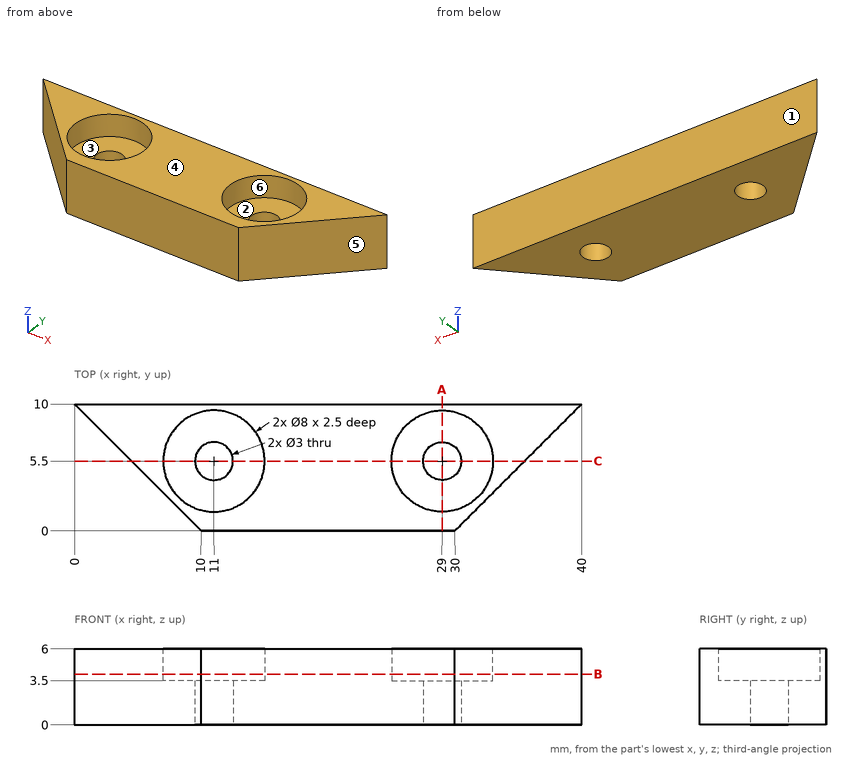
The drawing under review shows one solid part. Ordinate dimensions are in mm from its lowest x, y, z. A direction names the side the tool comes from. Coordinates: 2 decimals unless noted, no trailing zeros. Write each loop counter-clockwise with the first axis right and the second up, starting at its lowest first coordinate (ties: lowest second). Pieces come first, ordered by that corner, then holes. Notation, with made-up numbers: M 82,20 L 109,20 A24 ccw 109,44 Z; hole C 9,22 d7. An arc over 180 degrees is marked long. Put each result on its own line as item: value.
1) Add section B-B on z = 4. State how many separate pieces and enclosed holes the cut face has, then the cut area to 3 significant figures.
Computed:
separate pieces: 1
enclosed holes: 2
area: 199 mm2
2) Add section A-A on x = 29. Give the boundary of the cut face in (y, z), then the cut area to 3 significant figures.
Computed:
outline: M 0,0 L 4,0 L 4,3.5 L 1.5,3.5 L 1.5,6 L 0,6 Z; M 7,0 L 10,0 L 10,6 L 9.5,6 L 9.5,3.5 L 7,3.5 Z
area: 29.5 mm2
3) Draft analysis for pull direction Y (two halves, no side actions). For the marked faces 3, 4, 5 and 6, state which applies: released by +Y, released by -Y, zero draft, split by the parting line, or undercut.
Computed:
face 3: undercut
face 4: zero draft
face 5: released by -Y
face 6: undercut
4) Add section C-C on y = 5.5. Give the boundary of the cut face in (x, z).
Computed:
outline: M 4.5,0 L 9.5,0 L 9.5,3.5 L 7,3.5 L 7,6 L 4.5,6 Z; M 12.5,0 L 27.5,0 L 27.5,3.5 L 25,3.5 L 25,6 L 15,6 L 15,3.5 L 12.5,3.5 Z; M 30.5,0 L 35.5,0 L 35.5,6 L 33,6 L 33,3.5 L 30.5,3.5 Z
5) Wall thickness on probe 1 along Y at (x, z) = (11, 4.95); probe 2 along Y at (x, z) = (29, 1.55); probe 3 along X at (y, z) = (7.75, 4.25): over which ranges is each line inside the solid? List them lowest first. Write a range as [from, to].
Computed:
probe 1: y = [0, 1.5], [9.5, 10]
probe 2: y = [0, 4], [7, 10]
probe 3: x = [2.25, 7.69], [14.31, 25.69], [32.31, 37.75]
6) For the marked faces 1 and 2, list the 3-axis set-ups (+Z, -Z, +X, -X, +Y, -Y) from which the entire face can be reached by the end or side of a thin tool; tool diameter is ignored.
Computed:
face 1: +Z, -Z, +X, -X, +Y
face 2: +Z
7) Clearance check with flat-ended pins moving along their axes: pin 1 Ø2.5 at (x, y) = (27.5, 7.5) entering from +Z; pin 2 Ø2 at (y, z) = (5, 2) entering from -X. State where each tip first meets the part, or that it passes through.
Computed:
pin 1: stops at z = 3.5
pin 2: stops at x = 4
